Geometry check sheet. Reference: the model listing, model coordinates, mm. A direction names the side the tool comes from. Round coordinates to 2 decimals unless told otherwise and drop trailing zeros. Write each loop counter-clockwise with the first axis right and the second up, starting at its lowest first coordinate (ties: lowest second). Pieces come first, ordered by that corner, then holes. Notation, with made-up numbers: (-39, 55) - (20, 55) arc R16 ccw to (20, 81) - close; hole circle Ø8 at (5, 77.5). An arc over 180 degrees is marked (long way). Return JSON: item names as keys, results as strings.
```python
from build123d import *

# Parameters (mm, degrees)
EXTRUDE_1_DEPTH     = 1312
CUT_EXTRUDE_1_REACH = 17
SKETCH_2_R          = 25
CUT_EXTRUDE_2_REACH = 17
CUT_EXTRUDE_3_REACH = 17
SKETCH_4_R          = 7.5
SKETCH_4_R_2        = 12


with BuildPart() as part:
    # 스케치1 → 보스-돌출1 (new body)
    with BuildSketch(Plane(origin=(0, 0, 0), x_dir=(0, 0, -1), z_dir=(1, 0, 0))):
        Polygon((0, 0), (65, 0), (65, 1336), (50, 1336), (50, 6), (0, 6), align=None)
    extrude(amount=EXTRUDE_1_DEPTH)

    # 스케치2 → 컷-돌출1 (cut, up to next)
    with BuildSketch(Plane.XY.offset(-50), mode=Mode.PRIVATE) as cut_extrude_1_sk1:
        with Locations((656, 680)):
            Circle(SKETCH_2_R)
    cut_extrude_1_tool1 = extrude(cut_extrude_1_sk1.sketch, amount=-CUT_EXTRUDE_1_REACH, mode=Mode.PRIVATE) & part.part
    add(cut_extrude_1_tool1.solids().sort_by_distance((656, 680, -50))[0], mode=Mode.SUBTRACT)

    # 스케치3 → 컷-돌출2 (cut, up to next)
    with BuildSketch(Plane.XY.offset(-50), mode=Mode.PRIVATE) as cut_extrude_2_sk1:
        with BuildLine():
            ThreePointArc((0, 680), (192.137951542, 1143.862048458), (656, 1336))
            Line((656, 1336), (0, 1336))
            Line((0, 1336), (0, 680))
        make_face()
    cut_extrude_2_tool1 = extrude(cut_extrude_2_sk1.sketch, amount=-CUT_EXTRUDE_2_REACH, mode=Mode.PRIVATE) & part.part
    add(cut_extrude_2_tool1.solids().sort_by_distance((146.529368, 1189.470632, -50))[0], mode=Mode.SUBTRACT)
    # 스케치3 → 컷-돌출2 (cut, up to next)
    with BuildSketch(Plane.XY.offset(-50), mode=Mode.PRIVATE) as cut_extrude_2_sk2:
        with BuildLine():
            Line((1312, 680), (1312, 1336))
            Line((1312, 1336), (656, 1336))
            ThreePointArc((656, 1336), (1119.862048458, 1143.862048458), (1312, 680))
        make_face()
    cut_extrude_2_tool2 = extrude(cut_extrude_2_sk2.sketch, amount=-CUT_EXTRUDE_2_REACH, mode=Mode.PRIVATE) & part.part
    add(cut_extrude_2_tool2.solids().sort_by_distance((1165.470632, 1189.470632, -50))[0], mode=Mode.SUBTRACT)

    # 스케치4 → 컷-돌출3 (cut, up to next)
    with BuildSketch(Plane.XY.offset(-50), mode=Mode.PRIVATE) as cut_extrude_3_sk1:
        with Locations((25, 35)):
            Circle(SKETCH_4_R)
    cut_extrude_3_tool1 = extrude(cut_extrude_3_sk1.sketch, amount=-CUT_EXTRUDE_3_REACH, mode=Mode.PRIVATE) & part.part
    add(cut_extrude_3_tool1.solids().sort_by_distance((25, 35, -50))[0], mode=Mode.SUBTRACT)
    # 스케치4 → 컷-돌출3 (cut, up to next)
    with BuildSketch(Plane.XY.offset(-50), mode=Mode.PRIVATE) as cut_extrude_3_sk2:
        with Locations((25, 250)):
            Circle(SKETCH_4_R_2)
    cut_extrude_3_tool2 = extrude(cut_extrude_3_sk2.sketch, amount=-CUT_EXTRUDE_3_REACH, mode=Mode.PRIVATE) & part.part
    add(cut_extrude_3_tool2.solids().sort_by_distance((25, 250, -50))[0], mode=Mode.SUBTRACT)
    # 스케치4 → 컷-돌출3 (cut, up to next)
    with BuildSketch(Plane.XY.offset(-50), mode=Mode.PRIVATE) as cut_extrude_3_sk3:
        with Locations((25, 465)):
            Circle(SKETCH_4_R_2)
    cut_extrude_3_tool3 = extrude(cut_extrude_3_sk3.sketch, amount=-CUT_EXTRUDE_3_REACH, mode=Mode.PRIVATE) & part.part
    add(cut_extrude_3_tool3.solids().sort_by_distance((25, 465, -50))[0], mode=Mode.SUBTRACT)
    # 스케치4 → 컷-돌출3 (cut, up to next)
    with BuildSketch(Plane.XY.offset(-50), mode=Mode.PRIVATE) as cut_extrude_3_sk4:
        with Locations((25, 680)):
            Circle(SKETCH_4_R_2)
    cut_extrude_3_tool4 = extrude(cut_extrude_3_sk4.sketch, amount=-CUT_EXTRUDE_3_REACH, mode=Mode.PRIVATE) & part.part
    add(cut_extrude_3_tool4.solids().sort_by_distance((25, 680, -50))[0], mode=Mode.SUBTRACT)
    # 스케치4 → 컷-돌출3 (cut, up to next)
    with BuildSketch(Plane.XY.offset(-50), mode=Mode.PRIVATE) as cut_extrude_3_sk5:
        with Locations((73.032014985, 921.473245822)):
            Circle(SKETCH_4_R_2)
    cut_extrude_3_tool5 = extrude(cut_extrude_3_sk5.sketch, amount=-CUT_EXTRUDE_3_REACH, mode=Mode.PRIVATE) & part.part
    add(cut_extrude_3_tool5.solids().sort_by_distance((73.032015, 921.473246, -50))[0], mode=Mode.SUBTRACT)
    # 스케치4 → 컷-돌출3 (cut, up to next)
    with BuildSketch(Plane.XY.offset(-50), mode=Mode.PRIVATE) as cut_extrude_3_sk6:
        with Locations((209.815621071, 1126.184378929)):
            Circle(SKETCH_4_R_2)
    cut_extrude_3_tool6 = extrude(cut_extrude_3_sk6.sketch, amount=-CUT_EXTRUDE_3_REACH, mode=Mode.PRIVATE) & part.part
    add(cut_extrude_3_tool6.solids().sort_by_distance((209.815621, 1126.184379, -50))[0], mode=Mode.SUBTRACT)
    # 스케치4 → 컷-돌출3 (cut, up to next)
    with BuildSketch(Plane.XY.offset(-50), mode=Mode.PRIVATE) as cut_extrude_3_sk7:
        with Locations((414.526754178, 1262.967985015)):
            Circle(SKETCH_4_R_2)
    cut_extrude_3_tool7 = extrude(cut_extrude_3_sk7.sketch, amount=-CUT_EXTRUDE_3_REACH, mode=Mode.PRIVATE) & part.part
    add(cut_extrude_3_tool7.solids().sort_by_distance((414.526754, 1262.967985, -50))[0], mode=Mode.SUBTRACT)
    # 스케치4 → 컷-돌출3 (cut, up to next)
    with BuildSketch(Plane.XY.offset(-50), mode=Mode.PRIVATE) as cut_extrude_3_sk8:
        with Locations((656, 1311)):
            Circle(SKETCH_4_R_2)
    cut_extrude_3_tool8 = extrude(cut_extrude_3_sk8.sketch, amount=-CUT_EXTRUDE_3_REACH, mode=Mode.PRIVATE) & part.part
    add(cut_extrude_3_tool8.solids().sort_by_distance((656, 1311, -50))[0], mode=Mode.SUBTRACT)
    # 스케치4 → 컷-돌출3 (cut, up to next)
    with BuildSketch(Plane.XY.offset(-50), mode=Mode.PRIVATE) as cut_extrude_3_sk9:
        with Locations((897.473245822, 1262.967985015)):
            Circle(SKETCH_4_R_2)
    cut_extrude_3_tool9 = extrude(cut_extrude_3_sk9.sketch, amount=-CUT_EXTRUDE_3_REACH, mode=Mode.PRIVATE) & part.part
    add(cut_extrude_3_tool9.solids().sort_by_distance((897.473246, 1262.967985, -50))[0], mode=Mode.SUBTRACT)
    # 스케치4 → 컷-돌출3 (cut, up to next)
    with BuildSketch(Plane.XY.offset(-50), mode=Mode.PRIVATE) as cut_extrude_3_sk10:
        with Locations((1102.184378929, 1126.184378929)):
            Circle(SKETCH_4_R_2)
    cut_extrude_3_tool10 = extrude(cut_extrude_3_sk10.sketch, amount=-CUT_EXTRUDE_3_REACH, mode=Mode.PRIVATE) & part.part
    add(cut_extrude_3_tool10.solids().sort_by_distance((1102.184379, 1126.184379, -50))[0], mode=Mode.SUBTRACT)
    # 스케치4 → 컷-돌출3 (cut, up to next)
    with BuildSketch(Plane.XY.offset(-50), mode=Mode.PRIVATE) as cut_extrude_3_sk11:
        with Locations((1238.967985015, 921.473245822)):
            Circle(SKETCH_4_R_2)
    cut_extrude_3_tool11 = extrude(cut_extrude_3_sk11.sketch, amount=-CUT_EXTRUDE_3_REACH, mode=Mode.PRIVATE) & part.part
    add(cut_extrude_3_tool11.solids().sort_by_distance((1238.967985, 921.473246, -50))[0], mode=Mode.SUBTRACT)
    # 스케치4 → 컷-돌출3 (cut, up to next)
    with BuildSketch(Plane.XY.offset(-50), mode=Mode.PRIVATE) as cut_extrude_3_sk12:
        with Locations((1287, 680)):
            Circle(SKETCH_4_R_2)
    cut_extrude_3_tool12 = extrude(cut_extrude_3_sk12.sketch, amount=-CUT_EXTRUDE_3_REACH, mode=Mode.PRIVATE) & part.part
    add(cut_extrude_3_tool12.solids().sort_by_distance((1287, 680, -50))[0], mode=Mode.SUBTRACT)
    # 스케치4 → 컷-돌출3 (cut, up to next)
    with BuildSketch(Plane.XY.offset(-50), mode=Mode.PRIVATE) as cut_extrude_3_sk13:
        with Locations((1287, 465)):
            Circle(SKETCH_4_R_2)
    cut_extrude_3_tool13 = extrude(cut_extrude_3_sk13.sketch, amount=-CUT_EXTRUDE_3_REACH, mode=Mode.PRIVATE) & part.part
    add(cut_extrude_3_tool13.solids().sort_by_distance((1287, 465, -50))[0], mode=Mode.SUBTRACT)
    # 스케치4 → 컷-돌출3 (cut, up to next)
    with BuildSketch(Plane.XY.offset(-50), mode=Mode.PRIVATE) as cut_extrude_3_sk14:
        with Locations((1287, 250)):
            Circle(SKETCH_4_R_2)
    cut_extrude_3_tool14 = extrude(cut_extrude_3_sk14.sketch, amount=-CUT_EXTRUDE_3_REACH, mode=Mode.PRIVATE) & part.part
    add(cut_extrude_3_tool14.solids().sort_by_distance((1287, 250, -50))[0], mode=Mode.SUBTRACT)
    # 스케치4 → 컷-돌출3 (cut, up to next)
    with BuildSketch(Plane.XY.offset(-50), mode=Mode.PRIVATE) as cut_extrude_3_sk15:
        with Locations((1287, 35)):
            Circle(SKETCH_4_R_2)
    cut_extrude_3_tool15 = extrude(cut_extrude_3_sk15.sketch, amount=-CUT_EXTRUDE_3_REACH, mode=Mode.PRIVATE) & part.part
    add(cut_extrude_3_tool15.solids().sort_by_distance((1287, 35, -50))[0], mode=Mode.SUBTRACT)


solid = part.part
```
(1) Section check C-C, the plane x = 776. Enter the section's corners in (y, z).
Response values:
{"outline": "(0, -65) - (1324.93, -65) - (1324.93, -50) - (6, -50) - (6, 0) - (0, 0) - close"}
(2) Material ranges on line 1 along Z through (x, y) = (1220.5, 514); line 2 along Y through (x, z) = (532, -7.5); line 3 along Y through (x, z) = (382, -59), recorded low to high. Write a range as [from, to].
Response values:
{"line 1": "z = [-65, -50]", "line 2": "y = [0, 6]", "line 3": "y = [0, 1276.04]"}
(3) Release check for a two-part mould opening along X. For faces 3 (the face through (0, 342, -59)), 4 (the face through (647, 6, -25)), 5 (the face through (667.5, 657.8, -57.4)) record: pulls with the +X half, pulls with the -X half, needs draft (parallel to the pull), parting line crosses it, or undercut.
Response values:
{"face 3": "pulls with the -X half", "face 4": "needs draft", "face 5": "undercut"}
(4) Gauge pin test, flat ends, axial feed: pin 1 (1.5 mm diameter, centred on x = 769, y = 189.5, fed in from +Z); pin 2 (2 mm diameter, centred on x = 292.5, z = -40, fed in from +Y). Record the tip position at first contact, or that the pin passes through.
Response values:
{"pin 1": "stops at z = -50", "pin 2": "stops at y = 6"}
(5) Section check B-B, the plane y = 187.5. Enter the section's corners in (x, z).
Response values:
{"outline": "(0, -65) - (1312, -65) - (1312, -50) - (0, -50) - close"}
(6) Access from +Z, -Z, +X, -X, +Y, -Y to the whole of each face (thin tool, end or side, straight path). Record for faces 1 (the face through (647, 533, -50)), 2 (the face through (647, 0, -32)).
Response values:
{"face 1": "+Z, +X, -X, +Y", "face 2": "+Z, -Z, +X, -X, -Y"}
(7) Section check A-A, the plane z = -33. Enter the section's corners in (x, y), plus the area to 3 significant figures.
Response values:
{"outline": "(0, 0) - (1312, 0) - (1312, 6) - (0, 6) - close", "area": "7,870 mm^2"}
